Could you check a few things on this model? Use its own coordinates, in mm. A direction names the side the tool comes from. Coordinates: 2 decimals unless noted, no trailing zeros. Loops run counter-clockwise (first coordinate to the right, second up) from the corner with the lowest first, then second, coordinate; pieces in that order, holes last.
from build123d import *

# Parameters (mm, degrees)
F0_W      = 100
F0_H      = 100
F1_DEPTH  = 100
F3_R      = 10
F4_W      = 10
F4_H      = 10
F5_DEPTH  = 20
F6_R      = 7.5
F7_DEPTH  = 100.001
F10_DEPTH = 25
F11_SIZE  = 5


with BuildPart() as f1:
    # F0 (on Top) → F1 (new body)
    with BuildSketch(Plane.XY):
        with Locations((50, 50)):
            Rectangle(F0_W, F0_H)
    extrude(amount=F1_DEPTH)

    # F3
    f3_edges = [f1.edges().sort_by_distance(p)[0] for p in [
        (0, 50, 100),
    ]]
    fillet(f3_edges, radius=F3_R)

    # F4 (on face) → F5 (cut)
    with BuildSketch(Plane.XZ):
        with Locations((20, 15)):
            Rectangle(F4_W, F4_H)
        with Locations((40, 15)):
            Rectangle(F4_W, F4_H)
        with Locations((60, 15)):
            Rectangle(F4_W, F4_H)
        with Locations((80, 15)):
            Rectangle(F4_W, F4_H)
    extrude(amount=-F5_DEPTH, mode=Mode.SUBTRACT)

    # F6 (on face) → F7 (cut, through all)
    with BuildSketch(Plane.YZ.offset(100)):
        with Locations((50, 15)):
            Circle(F6_R)
    extrude(amount=-F7_DEPTH, mode=Mode.SUBTRACT)

    # F9 (on offset) → F10 (cut, symmetric)
    with BuildSketch(Plane.XZ.offset(-50)):
        Polygon((0, 90), (100, 50), (100, 100), (0, 100), align=None)
    extrude(amount=F10_DEPTH, both=True, mode=Mode.SUBTRACT)

    # F11
    f11_edges = [f1.edges().sort_by_distance(p)[0] for p in [
        (100, 0, 50),
        (100, 100, 50),
    ]]
    chamfer(f11_edges, length=F11_SIZE)


solid = f1.part
(1) We'd pull the mould along Y, two halves only. Please class faces 3 (the face through (60, 20, 15)), 4 (the face through (60, 75, 81)), 5 (the face through (65, 10, 15)): +Y half, -Y half, draft (parallel to the pull), parting line (faces both ways), or undercut.
Answers:
face 3: -Y half
face 4: undercut
face 5: draft
(2) Imagine slicing it at B-B, the plane x = 93. Write out the boundary of the cut face in (y, z), and give its area (3 significant figures).
Answers:
outline: (0, 0) - (100, 0) - (100, 100) - (75, 100) - (75, 52.8) - (25, 52.8) - (25, 100) - (0, 100) - close; hole circle Ø15 at (50, 15)
area: 7,460 mm2
(3) Imagine slicing it at D-D, the plane z = 80. Write out the boundary of the cut face in (x, y).
Answers:
outline: (0, 0) - (95, 0) - (100, 5) - (100, 25) - (25, 25) - (25, 75) - (100, 75) - (100, 95) - (95, 100) - (0, 100) - close
(4) I need wall thicknesses on probe 1 along Y at (x, z) = (32, 95.5); probe 2 along Z at (x, y) = (57, 50); probe 3 along Z at (x, y) = (14, 56). Which ranges of each line are inside material? Lowest first, please.
Answers:
probe 1: y = 0 to 25, 75 to 100
probe 2: z = 0 to 7.5, 22.5 to 67.2
probe 3: z = 0 to 10.5, 19.5 to 84.4
(5) Imagine slicing it at C-C, the plane y = 50. Write out the boundary of the cut face in (x, z).
Answers:
outline: (0, 0) - (100, 0) - (100, 7.5) - (0, 7.5) - close; (0, 22.5) - (100, 22.5) - (100, 50) - (0, 90) - close
(6) Imagine slicing it at A-A, the plane z = 15. Write out the boundary of the cut face in (x, y).
Answers:
outline: (0, 0) - (15, 0) - (15, 20) - (25, 20) - (25, 0) - (35, 0) - (35, 20) - (45, 20) - (45, 0) - (55, 0) - (55, 20) - (65, 20) - (65, 0) - (75, 0) - (75, 20) - (85, 20) - (85, 0) - (95, 0) - (100, 5) - (100, 42.5) - (0, 42.5) - close; (0, 57.5) - (100, 57.5) - (100, 95) - (95, 100) - (0, 100) - close
(7) Which directions (+Z, -Z, +X, -X, +Y, -Y) give clear straight access to the entire face, cutting with the end or side of a thin tool? Please do faces 1 (the face through (55, 10, 15)), 2 (the face through (2.85, 87.68, 96.99)).
Answers:
face 1: -Y
face 2: +Z, -X, +Y, -Y
(8) For pin 1 (3 mm diameter, centred on y = 57, z = 85, fed in from +X); pin 2 (12 mm diameter, centred on x = 57.5, y = 44.5, fed in from +Z), each with a flat end and sliding along its axis, tell me the tip position at first contact or that it passes through.
Answers:
pin 1: stops at x = 16.25
pin 2: stops at z = 69.4
